from build123d import *

# Parameters (mm, degrees)
CHAMFER1_SIZE           = 0.254
SKETCH2_W               = 7.0612
SKETCH2_H               = 0.762
CUT_EXTRUDE1_DEPTH      = 4.175
CUT_EXTRUDE1_DEPTH_BACK = 4.175


with BuildPart() as part:
    # Sketch1 → Revolve1 (revolve)
    with BuildSketch(Plane.XY, mode=Mode.PRIVATE) as revolve1_sk:
        with BuildLine():
            Line((1.9558, 3.175), (2.0828, 3.175))
            Line((2.0828, 3.175), (2.0828, 0.889))
            Line((2.0828, 0.889), (2.08534, 0.889))
            Line((2.08534, 0.889), (2.08534, 2.54))
            Line((2.08534, 2.54), (2.59334, 2.54))
            Line((2.59334, 2.54), (2.59334, 1.9685))
            Line((2.59334, 1.9685), (9.65454, 1.9685))
            Line((9.65454, 1.9685), (9.65454, 1.277822692))
            Line((9.65454, 1.277822692), (2.59334, 1.277822692))
            Line((2.59334, 1.277822692), (2.59334, 0))
            Line((2.59334, 0), (0, 0))
            ThreePointArc((0, 0), (0.528187929, 1.864522636), (1.9558, 3.175))
        make_face()
    revolve(revolve1_sk.sketch.rotate(Axis((0, 0, 0), (1, 0, 0)), 90), axis=Axis((0, 0, 0), (1, 0, 0)))  # turned: the seam where the file's is

    # Chamfer1
    chamfer1_edges = [part.edges().sort_by_distance(p)[0] for p in [
        (9.65454, 0, -1.9685),
    ]]
    chamfer(chamfer1_edges, length=CHAMFER1_SIZE)

    # Sketch2 → Cut-Extrude1 (cut, two sides)
    with BuildSketch(Plane.XY) as cut_extrude1_sk:
        with Locations((6.12394, 0)):
            Rectangle(SKETCH2_W, SKETCH2_H)
    extrude(amount=CUT_EXTRUDE1_DEPTH, mode=Mode.SUBTRACT)
    extrude(cut_extrude1_sk.sketch, amount=-CUT_EXTRUDE1_DEPTH_BACK, mode=Mode.SUBTRACT)


solid = part.part
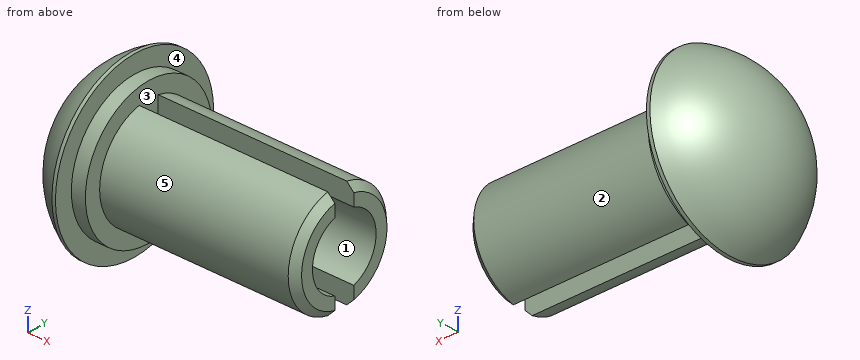
Work out the finished part from the listing and answer in its coordinate system (mm). Face numbers are marked on the shaded views. A direction names the side the tool comes from. Give positions to 0.01 mm unless a question says otherwise; leave off trailing zeros. Write each loop counter-clockwise with the first axis right and the second up, starting at its lowest first coordinate (ties: lowest second). Pieces come first, ordered by that corner, then holes. Notation, with made-up numbers: M 79,26 L 90,26 A29 ccw 90,54 Z; hole C 25.25,44 d11. An arc over 180 degrees is marked long. Answer as CSV lines item,"result".
Q1. The mould has two halves that part along Z. Classify the marked faces 1 and 2: +Z half, -Z half, draft (parallel to the pull), parting line (faces both ways), or undercut.
A:
face 1,"undercut"
face 2,"parting line"
Q2. Given P1, Ø0.8, axis at x = 4.5, z = -1.5, coming from the +Y side; P2, Ø1.5, axis at y = 1, z = -0.5, coming from the -X side; P3, Ø2, axis at x = 4.5, y = -0.5, coming from the -Z side; P4, Ø2, axis at x = 3, y = 0, coming from the +Z side (3 decimals), each flat-ended and moving along its own axis, determine where each tip first touches the part or whether it passes through.
A:
P1,"stops at y = 1.63"
P2,"stops at x = 0.02"
P3,"stops at z = -1.93"
P4,"stops at z = 3.175"
Q3. Find the intervals of material crossed by probe 1 along Y at (x, z) = (7.5, -1.5); probe 2 along Y at (x, z) = (2.25, 0); probe 3 along Z at (x, y) = (3, -1), in increasing order. Write a range as [from, to].
A:
probe 1,"y = [-1.27, -0.38], [0.38, 1.27]"
probe 2,"y = [-2.54, 2.54]"
probe 3,"z = [-1.7, -0.8], [0.8, 1.7]"
Q4. A tool of negligible diameter and unlimited length cuts with its end or side. For the marked faces 3, 4 and 5, from which of +Z, -Z, +X, -X, +Y, -Y can it reach the whole face along a straight path? Write none if from no direction.
A:
face 3,"+X"
face 4,"none"
face 5,"+X, -Y"
Q5. A cutting plane is placed at B-B on x = 9.25. Write down the section's boundary in (y, z), plus the area to 3 significant figures.
A:
outline,"M -0.38,-1.93 L -0.38,-1.22 A1.28 cw -0.38,1.22 L -0.38,1.93 A1.97 ccw Z; M 0.38,-1.93 A1.97 ccw 0.38,1.93 L 0.38,1.22 A1.28 cw 0.38,-1.22 Z"
area,"5.98 mm²"
